from build123d import *

# Parameters (mm, degrees)
F1_DEPTH    = 4
F2_DEPTH    = 14
F3_W        = 53.352586925
F3_H        = 25.252586925
F4_DEPTH    = 4
F3_W_2      = 25.252586925
F3_H_2      = 53.352586925
F5_DEPTH    = 4
F6_T4_DEPTH = 265.2829915773
F6_T9_DEPTH = 265.2829915773


# Not quite as in the source:
# - a fillet or chamfer that OpenCascade refuses, or shapes differently, is made with other operations: its cross-section is extruded or revolved along the edge and cut away or added


with BuildPart() as f1:
    # F0 (on Top) → F1 (new body)
    with BuildSketch(Plane.XY):
        with BuildLine():
            ThreePointArc((0, 125), (-14.05, 139.05), (-28.1, 125))
            Line((-28.1, 125), (0, 125))
        make_face()
        with BuildLine():
            Line((0, 125), (-28.1, 125))
            ThreePointArc((-28.1, 125), (-14.05, 110.95), (0, 125))
        make_face()
        with BuildLine():
            Line((-28.1, 125), (-28.1, 116.1781181146))
            ThreePointArc((-28.1, 116.1781181146), (-14.05, 108.41), (0, 116.1781181146))
            Line((0, 116.1781181146), (0, 125))
            ThreePointArc((0, 125), (-14.05, 110.95), (-28.1, 125))
        make_face()
        with BuildLine():
            Line((-28.1, 0), (0, 0))
            Line((0, 0), (0, 28.1))
            Line((0, 28.1), (0, 116.1781181146))
            ThreePointArc((0, 116.1781181146), (-14.05, 108.41), (-28.1, 116.1781181146))
            Line((-28.1, 116.1781181146), (-28.1, 0))
        make_face()
        with BuildLine():
            Line((0, 28.1), (0, 0))
            Line((0, 0), (28.1, 0))
            Line((28.1, 0), (116.1781181146, 0))
            ThreePointArc((116.1781181146, 0), (108.41, 14.05), (116.1781181146, 28.1))
            Line((116.1781181146, 28.1), (0, 28.1))
        make_face()
        with BuildLine():
            ThreePointArc((139.05, 14.05), (134.9348502757, 23.9848502757), (125, 28.1))
            Line((125, 28.1), (125, 0))
            ThreePointArc((125, 0), (134.9348502757, 4.1151497243), (139.05, 14.05))
        make_face()
        with BuildLine():
            Line((125, 0), (125, 28.1))
            ThreePointArc((125, 28.1), (110.95, 14.05), (125, 0))
        make_face()
        with BuildLine():
            Line((28.1, 0), (0, 0))
            Line((0, 0), (0, -28.1))
            Line((0, -28.1), (0, -116.1781181146))
            ThreePointArc((0, -116.1781181146), (14.05, -108.41), (28.1, -116.1781181146))
            Line((28.1, -116.1781181146), (28.1, 0))
        make_face()
        with BuildLine():
            Line((28.1, -125), (0, -125))
            ThreePointArc((0, -125), (14.05, -139.05), (28.1, -125))
        make_face()
        with BuildLine():
            ThreePointArc((28.1, -125), (14.05, -110.95), (0, -125))
            Line((0, -125), (28.1, -125))
        make_face()
        with BuildLine():
            ThreePointArc((28.1, -116.1781181146), (14.05, -108.41), (0, -116.1781181146))
            Line((0, -116.1781181146), (0, -125))
            ThreePointArc((0, -125), (14.05, -110.95), (28.1, -125))
            Line((28.1, -125), (28.1, -116.1781181146))
        make_face()
        with BuildLine():
            Line((-125, -28.1), (-125, 0))
            ThreePointArc((-125, 0), (-139.05, -14.05), (-125, -28.1))
        make_face()
        with BuildLine():
            ThreePointArc((-110.95, -14.05), (-115.0651497243, -4.1151497243), (-125, 0))
            Line((-125, 0), (-125, -28.1))
            ThreePointArc((-125, -28.1), (-115.0651497243, -23.9848502757), (-110.95, -14.05))
        make_face()
        with BuildLine():
            ThreePointArc((-108.41, -14.05), (-110.4813375189, -6.0227626321), (-116.1781181146, 0))
            Line((-116.1781181146, 0), (-125, 0))
            ThreePointArc((-125, 0), (-115.0651497243, -4.1151497243), (-110.95, -14.05))
            ThreePointArc((-110.95, -14.05), (-115.0651497243, -23.9848502757), (-125, -28.1))
            Line((-125, -28.1), (-116.1781181146, -28.1))
            ThreePointArc((-116.1781181146, -28.1), (-110.4813375189, -22.0772373679), (-108.41, -14.05))
        make_face()
        with BuildLine():
            Line((0, -28.1), (0, 0))
            Line((0, 0), (-28.1, 0))
            Line((-28.1, 0), (-116.1781181146, 0))
            ThreePointArc((-116.1781181146, 0), (-110.4813375189, -6.0227626321), (-108.41, -14.05))
            ThreePointArc((-108.41, -14.05), (-110.4813375189, -22.0772373679), (-116.1781181146, -28.1))
            Line((-116.1781181146, -28.1), (0, -28.1))
        make_face()
        with BuildLine():
            Line((125, 28.1), (116.1781181146, 28.1))
            ThreePointArc((116.1781181146, 28.1), (108.41, 14.05), (116.1781181146, 0))
            Line((116.1781181146, 0), (125, 0))
            ThreePointArc((125, 0), (110.95, 14.05), (125, 28.1))
        make_face()
    extrude(amount=F1_DEPTH)

    # F0 (on Top) → F2 (join)
    with BuildSketch(Plane.XY):
        with BuildLine():
            ThreePointArc((2.54, 125), (-18.6401307171, 140.9423586712), (-28.1, 116.1781181146))
            Line((-28.1, 116.1781181146), (-28.1, 125))
            ThreePointArc((-28.1, 125), (-14.05, 139.05), (0, 125))
            Line((0, 125), (0, 116.1781181146))
            ThreePointArc((0, 116.1781181146), (1.8923586712, 120.4098692829), (2.54, 125))
        make_face()
        with BuildLine():
            ThreePointArc((141.59, 14.05), (133.0272373679, 28.5686624811), (116.1781181146, 28.1))
            Line((116.1781181146, 28.1), (125, 28.1))
            ThreePointArc((125, 28.1), (134.9348502757, 23.9848502757), (139.05, 14.05))
            ThreePointArc((139.05, 14.05), (134.9348502757, 4.1151497243), (125, 0))
            Line((125, 0), (116.1781181146, 0))
            ThreePointArc((116.1781181146, 0), (133.0272373679, -0.4686624811), (141.59, 14.05))
        make_face()
        with BuildLine():
            Line((0, -125), (0, -116.1781181146))
            ThreePointArc((0, -116.1781181146), (9.4598692829, -140.9423586712), (30.64, -125))
            ThreePointArc((30.64, -125), (29.9923586712, -120.4098692829), (28.1, -116.1781181146))
            Line((28.1, -116.1781181146), (28.1, -125))
            ThreePointArc((28.1, -125), (14.05, -139.05), (0, -125))
        make_face()
        with BuildLine():
            Line((-125, 0), (-116.1781181146, 0))
            ThreePointArc((-116.1781181146, 0), (-141.59, -14.05), (-116.1781181146, -28.1))
            Line((-116.1781181146, -28.1), (-125, -28.1))
            ThreePointArc((-125, -28.1), (-139.05, -14.05), (-125, 0))
        make_face()
    extrude(amount=F2_DEPTH)

    # F3 (on face) → F4 (join)
    with BuildSketch(Plane.XY.offset(4)):
        with Locations((26.6762934625, 40.7262934625)):
            Rectangle(F3_W, F3_H)
    extrude(amount=-F4_DEPTH)

    # F3 (on face) → F5 (join)
    with BuildSketch(Plane.XY.offset(4)):
        with Locations((40.7262934625, -26.6762934625)):
            Rectangle(F3_W_2, F3_H_2)
        with Locations((-26.6762934625, -40.7262934625)):
            Rectangle(F3_W, F3_H)
        with Locations((-40.7262934625, 26.6762934625)):
            Rectangle(F3_W_2, F3_H_2)
    extrude(amount=-F5_DEPTH)

    # F6: chamfer of 50.8 on 2 edges, made by hand


with BuildPart() as f6_tool2:
    # F6_s3 → F6_t4 (new body)
    with BuildSketch(Plane.XY.offset(134.6414957887)):
        Polygon((2.552586925, -53.352586925), (53.352586925, -2.552586925), (53.352586925, -53.352586925), align=None)
    extrude(amount=-F6_T4_DEPTH)

    split(bisect_by=Plane.YZ.offset(28.1), keep=Keep.TOP)


with BuildPart() as f1_1:
    add(f1.part)

    # F6_t1: cut F6_tool2
    add(f6_tool2.part, mode=Mode.SUBTRACT)


with BuildPart() as f6_tool7:
    # F6_s8 → F6_t9 (new body)
    with BuildSketch(Plane.XY.offset(134.6414957887)):
        Polygon((-2.552586925, 53.352586925), (-53.352586925, 2.552586925), (-53.352586925, 53.352586925), align=None)
    extrude(amount=-F6_T9_DEPTH)

    split(bisect_by=Plane.YZ.offset(-28.1), keep=Keep.BOTTOM)


with BuildPart() as f1_2:
    add(f1_1.part)

    # F6_t6: cut F6_tool7
    add(f6_tool7.part, mode=Mode.SUBTRACT)


solid = f1_2.part
The model under review builds one solid part; all positions refer to its coordinate system, in mm. A direction names the side the tool comes from. Give positions to 0.01 mm unless a question says otherwise; leave off trailing zeros. Order: outer loops, then holes, each group sorted by start corner. A loop starts at its lowest first (then second) coordinate and runs counter-clockwise, first axis right, second up. Notation, with made-up numbers: M -38.75,74 L 6.25,74 A19 ccw 6.25,84 Z; hole C 18,28 d9. An arc over 180 degrees is marked long. Use one line per item in the form item = value. Start each with the question number.
Item 1: We need section C-C on y = 35.5. Give the boundary of the cut face in (x, z), plus the area to 3 significant figures.
Item 2: We need section A-A on z = 11.75. Give the boundary of the cut face in (x, y), plus the area to 3 significant figures.
Item 3: Insertion check: pin 1 Ø1.3 at (y, z) = (0.5, 3) entering from -X; pin 2 Ø2 at (y, z) = (-27, 8) entering from -X; pin 3 Ø3 at (y, z) = (-39, 1.5) entering from -X; pin 4 Ø1.5 at (x, y) = (15.5, -113) entering from -Z. Each pin has a flat end and moves straight along its axis. Give the tip position at first contact, or say it passes through.
Item 4: To check wall thickness, follow line 1 along Z through (x, y) = (18, -129.5); line 2 along X through (y, z) = (-13, 5.5); line 3 along X through (y, z) = (-68, 1.25). State the ranges of each line that lie inside material, in increasing order. Write a range as from..to.
Item 5: The part is to be moulded in two halves that separate along Y. For faces 1 (the flat face through (-14.1, 139.3, 14)), 2 (the flat face through (0, 121, 9)), 3 (the flat face through (121, 0, 9)), 4 (the cylindrical face through (-141.583, -13.555, 6.902)), say which applies: pulls with the +Y half, pulls with the -Y half, needs draft (parallel to the pull), parting line crosses it, or undercut.
Item 6: For faces 5 (the flat face through (121, 28.1, 9)), 6 (the flat face through (-121, 0, 9)), 7 (the flat face through (28.1, -121, 9)), 8 (the flat face through (-121, -28.1, 9)), list the 3-axis set-ups (+Z, -Z, +X, -X, +Y, -Y) from which the entire face can be reached by the end or side of a thin tool; tool diameter is ignored.
Item 7: We need section D-D on x = -78. Give the boundary of the cut face in (y, z).
Item 8: We need section B-B on x = 14.05. Give the boundary of the cut face in (y, z).
Completed:
q1.outline = M -28.1,0 L 53.35,0 L 53.35,4 L -28.1,4 Z
q1.area = 326 mm²
q2.outline = M -125,-28.1 A14.05 cw -125,0 L -116.18,0 A16.59 ccw long -116.18,-28.1 Z; M -28.1,116.18 L -28.1,125 A14.05 cw 0,125 L 0,116.18 A16.59 ccw long Z; M 0,-125 L 0,-116.18 A16.59 ccw long 28.1,-116.18 L 28.1,-125 A14.05 cw Z; M 116.18,0 A16.59 ccw long 116.18,28.1 L 125,28.1 A14.05 cw 125,0 Z
q2.area = 610 mm²
q3.pin_1 = -134.06
q3.pin_2 = -136.51
q3.pin_3 = -53.35
q3.pin_4 = 0
q4.line_1 = 0..4
q4.line_2 = -141.56..-139.01
q4.line_3 = 0..28.1
q5.face_1 = needs draft
q5.face_2 = undercut
q5.face_3 = undercut
q5.face_4 = parting line crosses it
q6.face_5 = +Z, -X
q6.face_6 = +Z
q6.face_7 = +Z, +Y
q6.face_8 = +Z, +X
q7.outline = M -28.1,0 L 0,0 L 0,4 L -28.1,4 Z
q8.outline = M -141.59,0 L 53.35,0 L 53.35,4 L -139.05,4 L -139.05,14 L -141.59,14 Z
